Autodesk Inventor part; units mm, degrees
ref_plane "YZ Plane" through (0, 0, 0) normal (1, 0, 0) x (0, 1, 0)
ref_plane "XZ Plane" through (0, 0, 0) normal (0, 1, 0) x (-1, 0, 0)
ref_plane "XY Plane" through (0, 0, 0) normal (0, 0, 1) x (1, 0, 0)
sketch "Sketch1" plane through (0, 0, 0) normal (0, 0, 1) x (1, 0, 0)
  line L0 (-31.9674, 70.0993) -> (31.9674, 70.0993)
  line L1 (31.9674, 70.0993) -> (31.9674, -74.8548)
  line L2 (31.9674, -74.8548) -> (-31.9674, -74.8548)
  line L3 (-31.9674, -74.8548) -> (-31.9674, 70.0993)
  circle A0 centre (-44.1203, 17.5249) radius 32.3435
  circle A1 centre (44.1203, 17.5249) radius 32.3435
  line L4 (0, 0) -> (0, 29.7658) construction
  line L5 (-44.1203, 17.5249) -> (44.1203, 17.5249)
  line L6 (44.1203, 17.5249) -> (44.1203, -17.5249)
  line L7 (44.1203, -17.5249) -> (-44.1203, -17.5249)
  line L8 (-44.1203, -17.5249) -> (-44.1203, 17.5249)
  line L9 (0, 0) -> (9.4229, 0) construction
  circle A2 centre (44.1203, -17.5249) radius 32.3435
  circle A3 centre (-44.1203, -17.5249) radius 32.3435
  line L10 (-11.7768, 40.2762) -> (11.7768, 40.2762)
  line L11 (11.7768, 40.2762) -> (11.7768, -36.31)
  line L12 (11.7768, -36.31) -> (-11.7768, -36.31)
  line L13 (-11.7768, -36.31) -> (-11.7768, 40.2762)
  point P0 (-31.9674, 47.4983)
  point P1 (-11.7768, 17.5249)
  point P2 (-11.7768, -17.5249)
  point P3 (-31.9674, -47.4983)
  point P4 (31.9674, -47.4983)
  point P5 (11.7768, -17.5249)
  point P6 (11.7768, 17.5249)
  point P7 (31.9674, 47.4983)
extrude "Extrusion1" add sketch "Sketch1" along normal blind 3.81 contours L0 L1 A1 L11 L10 L13 A0 L3 | L13 L10 L11 L5 | L5 L11 L7 L13 | L13 L12 L11 A2 L1 L2 L3 A3 | L7 L11 L12 L13
sketch "Sketch2" plane through (0, 0, 3.81) normal (0, 0, 1) x (1, 0, 0)
  line L0 (-20.9663, 30.173) -> (25.2183, 30.173)
  line L1 (25.2183, 30.173) -> (25.2183, -34.1474)
  line L2 (25.2183, -34.1474) -> (-20.9663, -34.1474)
  line L3 (-20.9663, -34.1474) -> (-20.9663, 30.173)
  point P0 (0, 0)
extrude "Extrusion2" cut sketch "Sketch2" against normal blind 0.0025
properties part number "dogbone" material "Speckle pattern"
Read the model definition and answer for the solid it produces. Units are mm, in the model's axes. A direction names the side the tool comes from. Coordinates: 2 decimals unless noted, no trailing zeros. Write each loop counter-clockwise with the first axis right and the second up, starting at its lowest first coordinate (ties: lowest second). Pieces come first, ordered by that corner, then holes. Notation, with made-up numbers: (41.25, -10) -> (71.25, -10) arc R22 cw to (71.25, 13) -> close; hole circle Ø9 at (53.5, 61). An arc over 180 degrees is marked (long way). Answer as a JSON object with one key per item and string values.
Q1. A tool of negligible diameter and unlimited length cuts with its end or side. For faces 5 (the flat face through (-11.777, 0, 2)), 6 (the flat face through (0, -1, 0)), 7 (the cylindrical face through (17.146, 35.371, 1.878)), from which of +Z, -Z, +X, -X, +Y, -Y can it reach the whole face along a straight path? Write none if from no direction.
The answers:
{"face 5": "+Z, -Z, -X", "face 6": "-Z, +X, -X, +Y, -Y", "face 7": "+Z, -Z, +X"}
Q2. Determine the mould class of faces 1 (the flat face through (11.777, 0, 2)), 2 (the flat face through (0, 70.099, 2)), 3 (the flat face through (-31.967, 59, 2)), 4 (the cylindrical face through (-17.45, 35.82, 1.88)) for opening direction Y: pulls with the +Y half, pulls with the -Y half, needs draft (parallel to the pull), parting line crosses it, or undercut.
The answers:
{"face 1": "undercut", "face 2": "pulls with the +Y half", "face 3": "needs draft", "face 4": "undercut"}
Q3. Flat-ended cylindrical pins translate along their axes: pin 1 Ø1.1 at (y, z) = (-7.5, 3) entering from -X; pin 2 Ø2 at (y, z) = (-17.5, 1) entering from +X. Find the tip coordinate at first contact, or state that the pin passes through.
The answers:
{"pin 1": "stops at x = -11.78", "pin 2": "stops at x = 11.79"}
Q4. The part is cut by section B-B on z = 1.6. Give the vertices of the cut face in (x, y).
The answers:
{"outline": "(-31.97, -74.85) -> (31.97, -74.85) -> (31.97, -47.5) arc R32.34 cw to (11.78, -17.52) -> (11.78, 17.52) arc R32.34 cw to (31.97, 47.5) -> (31.97, 70.1) -> (-31.97, 70.1) -> (-31.97, 47.5) arc R32.34 cw to (-11.78, 17.52) -> (-11.78, -17.52) arc R32.34 cw to (-31.97, -47.5) -> close"}
Q5. Consider line 1 (Z direction, x = 6, y = -12.5); line 2 (Y direction, x = 23.5, z = 2.9); line 3 (Y direction, x = -21.5, z = 3.05). Determine where each line is inside the solid, lowest interval first. Write a range as [from, to].
The answers:
{"line 1": "z = [0, 3.81]", "line 2": "y = [-74.85, -42.44], [42.44, 70.1]", "line 3": "y = [-74.85, -40.64], [40.64, 70.1]"}
Q6. The part is cut by section D-D on x = 20. Give the vertices of the cut face in (y, z), then the cut area to 3 significant figures.
The answers:
{"outline": "(-74.85, 0) -> (-39.07, 0) -> (-39.07, 3.81) -> (-74.85, 3.81) -> close; (39.07, 0) -> (70.1, 0) -> (70.1, 3.81) -> (39.07, 3.81) -> close", "area": "255 mm2"}
Q7. The part is cut by section A-A on x = 27.5. Give the vertices of the cut face in (y, z), then the cut area to 3 significant figures.
The answers:
{"outline": "(-74.85, 0) -> (-45.27, 0) -> (-45.27, 3.81) -> (-74.85, 3.81) -> close; (45.27, 0) -> (70.1, 0) -> (70.1, 3.81) -> (45.27, 3.81) -> close", "area": "207 mm2"}
Q8. The part is cut by section C-C on y = 5.5. Give the vertices of the cut face in (x, z), then the cut area to 3 significant figures.
The answers:
{"outline": "(-11.78, 0) -> (11.78, 0) -> (11.78, 3.81) -> (-11.78, 3.81) -> close", "area": "89.7 mm2"}
